from build123d import *

# Parameters (mm, degrees)
CROQUIS1_W              = 10
CROQUIS1_H              = 10
SALIENTE_EXTRUIR1_DEPTH = 1
SALIENTE_EXTRUIR2_START = 5
SALIENTE_EXTRUIR2_DEPTH = 10
REDONDEO2_R             = 1
REDONDEO3_R             = 1


with BuildPart() as part:
    # Croquis1 → Saliente-Extruir1 (new body)
    with BuildSketch(Plane.XY):
        Rectangle(CROQUIS1_W, CROQUIS1_H)
    extrude(amount=SALIENTE_EXTRUIR1_DEPTH)

    # Croquis2 → Saliente-Extruir2 (add, through all)
    with BuildSketch(Plane(origin=(0, 0, 0), x_dir=(0, 0, -1), z_dir=(1, 0, 0)).offset(SALIENTE_EXTRUIR2_START)):
        with BuildLine():
            Line((-1, 3.5), (-1, 2))
            ThreePointArc((-1, 2), (-3, 0), (-1, -2))
            Line((-1, -2), (-1, -3.5))
            ThreePointArc((-1, -3.5), (-4.5, 0), (-1, 3.5))
        make_face()
    extrude(amount=-SALIENTE_EXTRUIR2_DEPTH)

    # Redondeo2
    redondeo2_edges = [part.edges().sort_by_distance(p)[0] for p in [
        (0, 3.5, 1),
    ]]
    fillet(redondeo2_edges, radius=REDONDEO2_R)

    # Redondeo3
    redondeo3_edges = [part.edges().sort_by_distance(p)[0] for p in [
        (0, -3.5, 1),
    ]]
    fillet(redondeo3_edges, radius=REDONDEO3_R)


solid = part.part
Verification items for the finished model (mm, model axes). A direction names the side the tool comes from. Give positions to 0.01 mm unless a question says otherwise; leave off trailing zeros. Order: outer loops, then holes, each group sorted by start corner. A loop starts at its lowest first (then second) coordinate and runs counter-clockwise, first axis right, second up. Notation, with made-up numbers: M 32.25,8.5 L 77.25,8.5 A16 cw 77.25,35.5 Z; hole C 30,-5.75 d3. An arc over 180 degrees is marked long. Answer as a JSON object with one key per item and string values. Group by question number.
1) Mould release check, pull along Z, two halves, no side actions. Record for faces 3 (the face through (5, -0.1, 0.7)), 4 (the face through (0, 0, 1)), 5 (the face through (0.1, -0.1, 4.5)): released by +Z, released by -Z, zero draft, split by the parting line, or undercut.
2) Scan lines: line 1 along Z through (x, y) = (-3.75, 4.5); line 2 along Z through (x, y) = (0.5, -1.75); line 3 along Z through (x, y) = (4, -1.25). Record each from-to range of solid material in increasing order. Write a range as [from, to].
3) Cross-section at C-C (z = 2.8). Enter the section's corners in (x, y), then the cut area to 3 significant figures.
4) Cross-section at B-B (x = 2). Enter the section's corners in (y, z), then the cut area to 3 significant figures.
5) Cross-section at A-A (y = 0). Enter the section's corners in (x, z), then the cut area to 3 significant figures.
6) Access from +Z, -Z, +X, -X, +Y, -Y to the whole of each face (thin tool, end or side, straight path). Record for faces 1 (the face through (0, 0, 3)), 2 (the face through (-5, -0.1, 0.7)).
7) Depth check by flat-ended pin: pin 1 Ø0.7 at (x, y) = (1.5, -5) entering from +Z; pin 2 Ø1 at (x, z) = (-3, 2) entering from +Y. Enter the tip coordinate at first touch or a pass-through.
Result sheet:
{
 "1": {"face 3": "zero draft", "face 4": "undercut", "face 5": "released by +Z"},
 "2": {"line 1": "z = [0, 1]", "line 2": "z = [0, 1], [1.97, 4.03]", "line 3": "z = [0, 1], [2.56, 4.27]"},
 "3": {"outline": "M -5,-3 L 5,-3 L 5,-0.87 L -5,-0.87 Z; M -5,0.87 L 5,0.87 L 5,3 L -5,3 Z", "area": "42.6 mm2"},
 "4": {"outline": "M -5,0 L 5,0 L 5,1 L 4.39,1 A1 cw 3.41,1.78 A3.5 ccw -3.41,1.78 A1 cw -4.39,1 L -5,1 Z; hole M -2,1 L 2,1 A2 ccw Z", "area": "23.3 mm2"},
 "5": {"outline": "M -5,0 L 5,0 L 5,1 L -5,1 Z; M -5,3 L 5,3 L 5,4.5 L -5,4.5 Z", "area": "25.0 mm2"},
 "6": {"face 1": "+X, -X", "face 2": "+Z, -Z, -X, +Y, -Y"},
 "7": {"pin 1": "stops at z = 1", "pin 2": "stops at y = 3.52"}
}
